CAD build for the part. Positions are in the model's coordinates, mm. Give positions to 0.01 mm unless a question says otherwise; leave off trailing zeros. Write each loop counter-clockwise with the first axis right and the second up, starting at its lowest first coordinate (ties: lowest second). Pieces come first, ordered by that corner, then holes. Notation, with made-up numbers: (-38, 2.5) -> (-6, 2.5) arc R16 ccw to (-6, 10.5) -> close; hole circle Ø5 at (3.25, 46). An arc over 180 degrees is marked (long way). Use one line per item in the form item = value. Start each with the question number.
from build123d import *

# Parameters (mm, degrees)
F0_R     = 1.5
F1_DEPTH = 1


with BuildPart() as f1:
    # F0 (on Top) → F1 (new body)
    with BuildSketch(Plane.XY):
        with BuildLine():
            Line((-17.494214, -18), (17.494214, -18))
            ThreePointArc((17.494214, -18), (17.851859, -17.851859), (18, -17.494214))
            Line((18, -17.494214), (18, -14.173142))
            ThreePointArc((18, -14.173142), (17.851859, -13.815498), (17.494214, -13.667356))
            Line((17.494214, -13.667356), (9.165291, -13.667356))
            ThreePointArc((9.165291, -13.667356), (5.629757, -12.20289), (4.165291, -8.667356))
            Line((4.165291, -8.667356), (4.165291, 8.667356))
            ThreePointArc((4.165291, 8.667356), (5.629757, 12.20289), (9.165291, 13.667356))
            Line((9.165291, 13.667356), (17.494214, 13.667356))
            ThreePointArc((17.494214, 13.667356), (17.851859, 13.815498), (18, 14.173142))
            Line((18, 14.173142), (18, 17.494214))
            ThreePointArc((18, 17.494214), (17.851859, 17.851859), (17.494214, 18))
            Line((17.494214, 18), (-17.494214, 18))
            ThreePointArc((-17.494214, 18), (-17.851859, 17.851859), (-18, 17.494214))
            Line((-18, 17.494214), (-18, 14.173142))
            ThreePointArc((-18, 14.173142), (-17.851859, 13.815498), (-17.494214, 13.667356))
            Line((-17.494214, 13.667356), (-9.165291, 13.667356))
            ThreePointArc((-9.165291, 13.667356), (-5.629757, 12.20289), (-4.165291, 8.667356))
            Line((-4.165291, 8.667356), (-4.165291, -8.667356))
            ThreePointArc((-4.165291, -8.667356), (-5.629757, -12.20289), (-9.165291, -13.667356))
            Line((-9.165291, -13.667356), (-17.494214, -13.667356))
            ThreePointArc((-17.494214, -13.667356), (-17.851859, -13.815498), (-18, -14.173142))
            Line((-18, -14.173142), (-18, -17.494214))
            ThreePointArc((-18, -17.494214), (-17.851859, -17.851859), (-17.494214, -18))
        make_face()
        with Locations((-16, -16)):
            Circle(F0_R, mode=Mode.SUBTRACT)
        with Locations((16, -16)):
            Circle(F0_R, mode=Mode.SUBTRACT)
        with Locations((-16, 16)):
            Circle(F0_R, mode=Mode.SUBTRACT)
        with Locations((16, 16)):
            Circle(F0_R, mode=Mode.SUBTRACT)
    extrude(amount=F1_DEPTH)


solid = f1.part
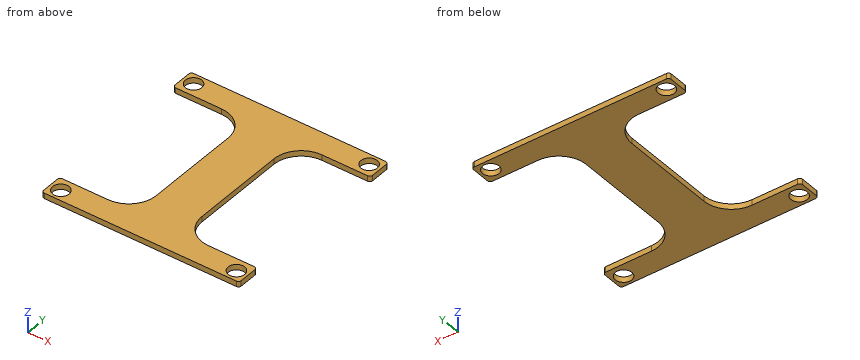
1) Cut at A-A (x = -16). Give the cut face in (y, z), and give its area (3 significant figures).
2) Cut at C-C (y = 16). Give the cut face in (x, z).
3) Cut at D-D (y = -15). Give the cut face in (x, z).
4) Cut at B-B (z = 0.3). Give the cut face in (x, y), and give its area (3 significant figures).
5) Wall check: line 1 along Y through (x, z) = (16, 0.2); line 2 along X through (y, z) = (15, 0.35); line 3 along Y through (x, z) = (16.5, 0.5). Give the ranges that are in metal, low to high. Write a range as from..to.
Final values:
q1.outline = (-18, 0) -> (-17.5, 0) -> (-17.5, 1) -> (-18, 1) -> close; (-14.5, 0) -> (-13.67, 0) -> (-13.67, 1) -> (-14.5, 1) -> close; (13.67, 0) -> (14.5, 0) -> (14.5, 1) -> (13.67, 1) -> close; (17.5, 0) -> (18, 0) -> (18, 1) -> (17.5, 1) -> close
q1.area = 2.67 mm^2
q2.outline = (-18, 0) -> (-17.5, 0) -> (-17.5, 1) -> (-18, 1) -> close; (-14.5, 0) -> (14.5, 0) -> (14.5, 1) -> (-14.5, 1) -> close; (17.5, 0) -> (18, 0) -> (18, 1) -> (17.5, 1) -> close
q3.outline = (-18, 0) -> (-17.12, 0) -> (-17.12, 1) -> (-18, 1) -> close; (-14.88, 0) -> (14.88, 0) -> (14.88, 1) -> (-14.88, 1) -> close; (17.12, 0) -> (18, 0) -> (18, 1) -> (17.12, 1) -> close
q4.outline = (-18, -17.49) arc R0.51 ccw to (-17.49, -18) -> (17.49, -18) arc R0.51 ccw to (18, -17.49) -> (18, -14.17) arc R0.51 ccw to (17.49, -13.67) -> (9.17, -13.67) arc R5 cw to (4.17, -8.67) -> (4.17, 8.67) arc R5 cw to (9.17, 13.67) -> (17.49, 13.67) arc R0.51 ccw to (18, 14.17) -> (18, 17.49) arc R0.51 ccw to (17.49, 18) -> (-17.49, 18) arc R0.51 ccw to (-18, 17.49) -> (-18, 14.17) arc R0.51 ccw to (-17.49, 13.67) -> (-9.17, 13.67) arc R5 cw to (-4.17, 8.67) -> (-4.17, -8.67) arc R5 cw to (-9.17, -13.67) -> (-17.49, -13.67) arc R0.51 ccw to (-18, -14.17) -> close; hole circle Ø3 at (-16, -16); hole circle Ø3 at (-16, 16); hole circle Ø3 at (16, -16); hole circle Ø3 at (16, 16)
q4.area = 532 mm^2
q5.line_1 = -18..-17.5, -14.5..-13.67, 13.67..14.5, 17.5..18
q5.line_2 = -18..-17.12, -14.88..14.88, 17.12..18
q5.line_3 = -18..-17.41, -14.59..-13.67, 13.67..14.59, 17.41..18
